Could you check a few things on this drawing? It's one solid part, dimensions in mm from its lowest x, y, z. Round coordinates to 2 decimals unless told otherwise and drop trailing zeros. Order: outer loops, then holes, each group sorted by start corner. A loop starts at its lowest first (then second) coordinate and runs counter-clockwise, first axis right, second up. Notation, with made-up numbers: (16.5, -38.75) - (40.5, -38.75) arc R20 cw to (40.5, -16.75) - close; hole circle Ø5 at (-6.75, -4). An arc over 180 degrees is marked (long way). Use one line per item in the form item = value.
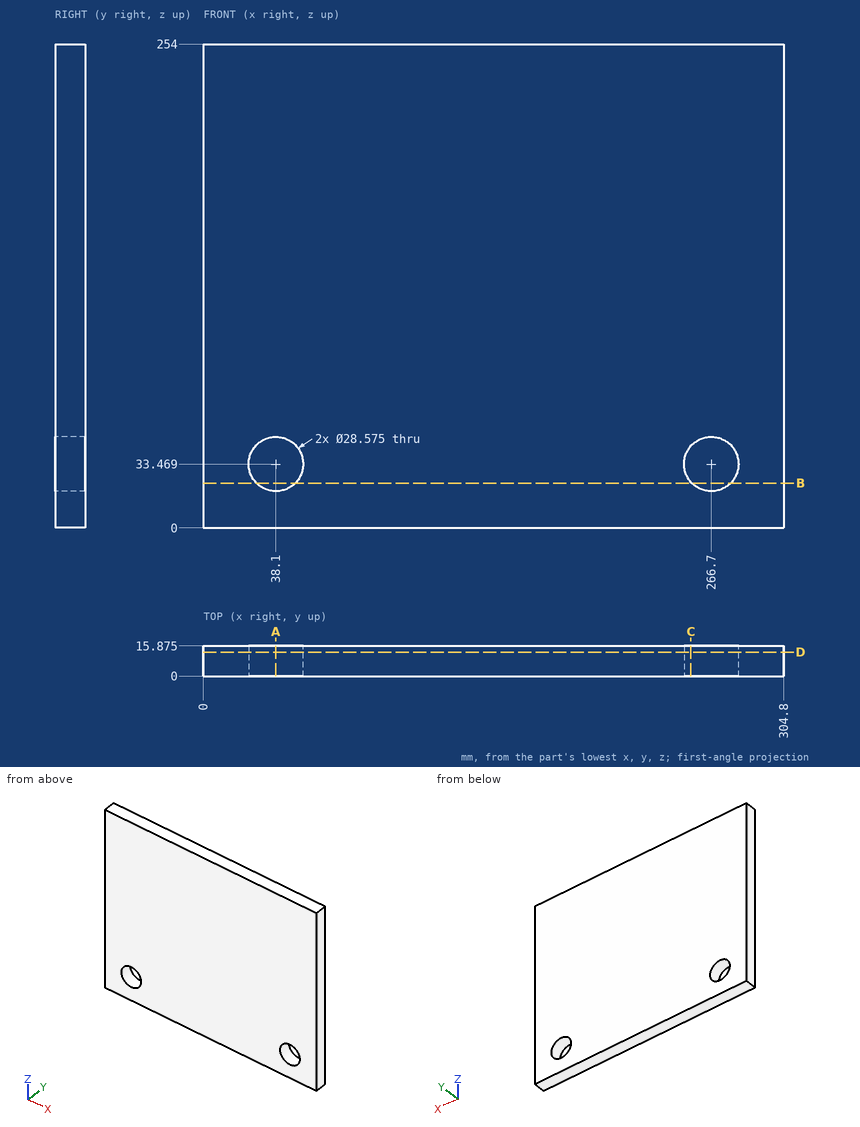
Item 1: Imagine slicing it at D-D on y = 12.5. Please give me the cut outline in (x, z) (1 decimal), plus the area to 3 significant figures.
Found:
outline = (0, 0) - (304.8, 0) - (304.8, 254) - (0, 254) - close; hole circle Ø28.6 at (38.1, 33.5); hole circle Ø28.6 at (266.7, 33.5)
area = 76,100 mm2
Item 2: Imagine slicing it at B-B on z = 23.5. Please give me the cut outline in (x, y) (1 decimal), plus the area to 3 significant figures.
Found:
outline = (0, 0) - (27.9, 0) - (27.9, 15.9) - (0, 15.9) - close; (48.3, 0) - (256.5, 0) - (256.5, 15.9) - (48.3, 15.9) - close; (276.9, 0) - (304.8, 0) - (304.8, 15.9) - (276.9, 15.9) - close
area = 4,190 mm2
Item 3: Imagine slicing it at A-A on x = 38.1. Please give me the cut outline in (y, z) (1 decimal).
Found:
outline = (0, 0) - (15.9, 0) - (15.9, 19.2) - (0, 19.2) - close; (0, 47.8) - (15.9, 47.8) - (15.9, 254) - (0, 254) - close
Item 4: I need wall thicknesses on L1, parallel to Z at x = 266.7, y = 8.5; L2, parallel to X at y = 12.5, z = 44 (1 decimal); L3, parallel to X at y = 11.5, z = 40. Which ranges of each line are inside material? Lowest first, please.
Found:
L1 = 0 to 19.18, 47.76 to 254
L2 = 0 to 28.4, 47.8 to 257, 276.4 to 304.8
L3 = 0 to 25.39, 50.81 to 253.99, 279.41 to 304.8
Item 5: Imagine slicing it at C-C on x = 256. Please give me the cut outline in (y, z) (1 decimal), plus the area to 3 significant figures.
Found:
outline = (0, 0) - (15.9, 0) - (15.9, 24) - (0, 24) - close; (0, 42.9) - (15.9, 42.9) - (15.9, 254) - (0, 254) - close
area = 3,730 mm2
